Here's how the part is built. I have some questions about the finished solid (model axes, mm). Face numbers are marked on the shaded views. A direction names the side the tool comes from. Give positions to 0.01 mm unless a question says otherwise; leave off trailing zeros. Loops run counter-clockwise (first coordinate to the right, second up) from the corner with the lowest first, then second, coordinate; pieces in that order, holes last. Notation, with made-up numbers: (41.5, 3) - (48.5, 3) arc R20 cw to (48.5, 27) - close; hole circle Ø10 at (-23.75, -14.75). An arc over 180 degrees is marked (long way). Use a Markdown table: item, result.
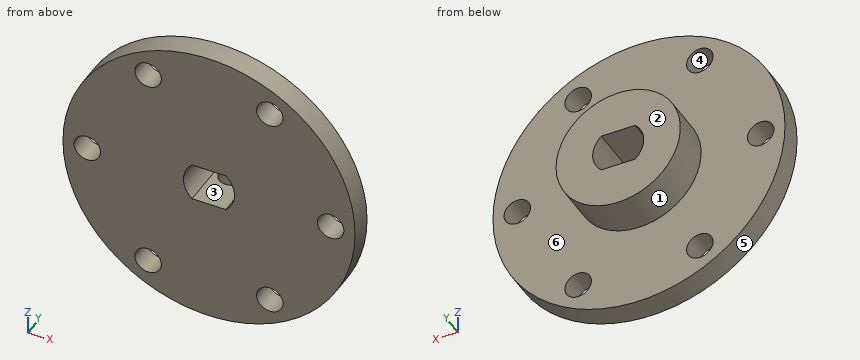
Autodesk Inventor part; units mm, degrees
ref_plane "YZ Plane" through (0, 0, 0) normal (1, 0, 0) x (0, 1, 0)
ref_plane "XZ Plane" through (0, 0, 0) normal (0, 1, 0) x (-1, 0, 0)
ref_plane "XY Plane" through (0, 0, 0) normal (0, 0, 1) x (1, 0, 0)
sketch "Sketch1" plane through (0, 0, 0) normal (0, 1, 0) x (-1, 0, 0)
  circle A0 centre (0, 0) radius 28.575
  circle A1 centre (0, 0) radius 23.8125 construction
  circle A2 centre (23.8125, 0) radius 2.5908
  circle A3 centre (0, 0) radius 28.575
  circle A4 centre (11.9063, 20.6222) radius 2.5908
  circle A5 centre (0, 0) radius 28.575
  circle A6 centre (-11.9062, 20.6222) radius 2.5908
  circle A7 centre (0, 0) radius 28.575
  circle A8 centre (-23.8125, 0) radius 2.5908
  circle A9 centre (0, 0) radius 28.575
  circle A10 centre (-11.9063, -20.6222) radius 2.5908
  circle A11 centre (0, 0) radius 28.575
  circle A12 centre (11.9062, -20.6222) radius 2.5908
  line L0 (-3.3001, 3.7528) -> (3.3001, 3.7528)
  line L1 (-3.3001, -3.7528) -> (3.3001, -3.7528)
  arc A13 (-3.3001, 3.7528) -> (-3.3001, -3.7528) centre (0, 0) ccw
  arc A14 (3.3001, -3.7528) -> (3.3001, 3.7528) centre (0, 0) ccw
  dimension "d1" = 47.625
  dimension "d0" = 57.15
  dimension "d2" = 5.1816
  dimension "d5" = 360
  dimension "d8" = 7.5057
  dimension "d9" = 3.7529
extrude "Extrusion1" add sketch "Sketch1" along normal blind 4.572
sketch "Sketch2" plane through (0, 4.572, 0) normal (0, 1, 0) x (1, 0, 0)
  arc A0 (-3.3001, 3.7528) -> (-3.3001, -3.7528) centre (0, 0) ccw
  line L0 (-3.3001, 3.7528) -> (3.3001, 3.7528)
  arc A1 (3.3001, -3.7528) -> (3.3001, 3.7528) centre (0, 0) ccw
  line L1 (3.3001, -3.7528) -> (-3.3001, -3.7528)
  circle A2 centre (0, 0) radius 28.575
  circle A3 centre (0, 0) radius 12.1666
  dimension "d12" = 24.3332
extrude "Extrusion2" add sketch "Sketch2" along normal blind 7.874 contours A3
sketch "Sketch3" plane through (-3.3001, 0, -3.7528) normal (0, 0, 1) x (1, 0, 0)
  line L0 (6.6002, 0) -> (6.6002, 12.446)
  line L1 (0, 12.446) -> (6.6002, 12.446)
  circle A0 centre (3.3001, 8.636) radius 2.413
  point P0 (3.3001, 0)
  dimension "d16" = 4.826
  dimension "d17" = 3.81
  dimension "d18" = 3.3001
extrude "Extrusion3" cut sketch "Sketch3" against normal blind 7.874
properties part number "Snow Blower Hub" material "Aluminum 6061"
(1) On a 3-axis mill with a long thin cutter (end or side, diameter ignored), from which of +Z, -Z, +X, -X, +Y, -Y can I reach the whole of each face in a straight line? I mean the marked faces 1, 2 and 3. Say none if no direction works.
A:
| item | result |
|---|---|
| face 1 | +Y |
| face 2 | +Z, -Z, +X, -X, +Y |
| face 3 | +Y, -Y |
(2) Will these pins go through, and if not, where does the flat tip stop? pin 1 (8.5 mm diameter, centred on x = -11.91, z = -20.62, fed in from +Y); pin 2 (4 mm diameter, centred on x = 0.5, y = 9, fed in from +Z); pin 3 (6 mm diameter, centred on y = 1.5, z = -9, fed in from -X); pin 4 (10 mm diameter, centred on x = -11, z = 5.5, fed in from +Y).
A:
| item | result |
|---|---|
| pin 1 | y = 4.57 |
| pin 2 | z = 12.17 |
| pin 3 | x = -27.94 |
| pin 4 | y = 12.45 |
(3) If I drill on line 1 (Y direction, x = -11.5, z = 12.5); line 2 (X direction, y = 4.25, z = -21); line 3 (X direction, y = 4.5, z = -2), over which ranges is the centre line in solid material (lowest first)?
A:
| item | result |
|---|---|
| line 1 | 0 to 4.57 |
| line 2 | -19.38 to -14.47, -9.34 to 9.34, 14.47 to 19.38 |
| line 3 | -28.5 to -25.46, -22.17 to -4.58, 4.58 to 22.17, 25.46 to 28.5 |
(4) Suppose I cut it at A-A on x = 0. Write out the boundary of the cut face in (y, z) (3 decimals), plus the area to 3 significant figures.
A:
| item | result |
|---|---|
| outline | (0, -28.575) - (4.572, -28.575) - (4.572, -12.167) - (12.446, -12.167) - (12.446, -3.753) - (11.049, -3.753) - (11.049, -11.627) - (6.223, -11.627) - (6.223, -3.753) - (0, -3.753) - close; (0, 3.753) - (12.446, 3.753) - (12.446, 12.167) - (4.572, 12.167) - (4.572, 28.575) - (0, 28.575) - close |
| area | 321 mm2 |
(5) We'd pull the mould along X, two halves only. Please class the marked faces 4, 5 and 6: pulls with the +X half, pulls with the -X half, needs draft (parallel to the pull), parting line crosses it, or undercut.
A:
| item | result |
|---|---|
| face 4 | undercut |
| face 5 | parting line crosses it |
| face 6 | needs draft |
(6) Suppose I cut it at D-D on x = -10. Write out the boundary of the cut face in (y, z), plus the area to 3 significant figures.
A:
| item | result |
|---|---|
| outline | (0, -26.77) - (4.57, -26.77) - (4.57, -22.38) - (0, -22.38) - close; (0, -18.87) - (4.57, -18.87) - (4.57, -6.93) - (12.45, -6.93) - (12.45, 6.93) - (4.57, 6.93) - (4.57, 18.87) - (0, 18.87) - close; (0, 22.38) - (4.57, 22.38) - (4.57, 26.77) - (0, 26.77) - close |
| area | 322 mm2 |
(7) Suppose I cut it at B-B on z = 0. Write out the boundary of the cut face in (x, y) (3 decimals), plus the area to 3 significant figures.
A:
| item | result |
|---|---|
| outline | (-28.575, 0) - (-26.403, 0) - (-26.403, 4.572) - (-28.575, 4.572) - close; (-21.222, 0) - (-4.997, 0) - (-4.997, 12.446) - (-12.167, 12.446) - (-12.167, 4.572) - (-21.222, 4.572) - close; (4.997, 0) - (21.222, 0) - (21.222, 4.572) - (12.167, 4.572) - (12.167, 12.446) - (4.997, 12.446) - close; (26.403, 0) - (28.575, 0) - (28.575, 4.572) - (26.403, 4.572) - close |
| area | 281 mm2 |
(8) Suppose I cut it at C-C on y = 10. Write out the boundary of the cut face in (x, z), plus the area to 3 significant figures.
A:
| item | result |
|---|---|
| outline | circle Ø24.33 at (0, 0); hole (-3.3, -3.75) - (-1.99, -3.75) - (-1.99, -11.63) - (1.99, -11.63) - (1.99, -3.75) - (3.3, -3.75) arc R5 ccw to (3.3, 3.75) - (-3.3, 3.75) arc R5 ccw to start |
| area | 366 mm2 |
